from build123d import *

# Parameters (mm, degrees)
F0_R     = 5.5
F0_R_2   = 4.1
F1_DEPTH = 16
F0_R_3   = 2.55
F2_DEPTH = 5
F3_SIZE  = 1
F4_R     = 0.75


with BuildPart() as f1:
    # F0 (on Top) → F1 (new body)
    with BuildSketch(Plane.XY):
        Circle(F0_R)
        Circle(F0_R_2, mode=Mode.SUBTRACT)
    extrude(amount=F1_DEPTH)

    # F0 (on Top) → F2 (join)
    with BuildSketch(Plane.XY):
        Circle(F0_R_2)
        Circle(F0_R_3, mode=Mode.SUBTRACT)
    extrude(amount=F2_DEPTH)

    # F3
    f3_edges = [f1.edges().sort_by_distance(p)[0] for p in [
        (-5.5, 0, 0),
    ]]
    chamfer(f3_edges, length=F3_SIZE)

    # F4 (on Front) → F5 (revolve, cut)
    with BuildSketch(Plane.XZ):
        with Locations((5.526415, 5.650808)):
            Circle(F4_R)
    revolve(axis=Axis((0, 0, 0), (0, 0, -1)), mode=Mode.SUBTRACT)


solid = f1.part
Check sheet for the modelled part. Datum: model origin and axes. Units: mm. A direction names the side the tool comes from. Give positions to 0.01 mm unless a question says otherwise; leave off trailing zeros. Loops run counter-clockwise (first coordinate to the right, second up) from the corner with the lowest first, then second, coordinate; pieces in that order, holes last. Notation, with made-up numbers: M 34.25,84.5 L 43.25,84.5 A29 ccw 43.25,118.5 Z; hole C 25.25,55 d7. An arc over 180 degrees is marked long. Return JSON: item names as keys, results as strings. Group by question number.
1. Cross-section at D-D on z = 6. Record the boundary of the cut face in (x, y), plus the area to 3 significant figures.
2. Tool access check on faces 4 (the cylindrical face through (-1.19, -5.37, 2.92)), 5 (the flat face through (-2, -2, 5)). Record the directions out of +Z, -Z, +X, -X, +Y, -Y that give a thin tool (end or side, any length) a straight path to the whole face; none if there is none.
3. Mould release check, pull along Y, two halves, no side actions. Record for faces 1 (the cylindrical face through (-1.19, -5.37, 11.13)), 2 (the cylindrical face through (-0.534, 4.065, 10.423)), 3 (the flat face through (2, -2, 0)): released by +Y, released by -Y, zero draft, split by the parting line, or undercut.
4. Cross-section at A-A on y = 0. Record the boundary of the cut face in (x, z).
5. Thickness scan on L1, parallel to Y at x = 0, z = 9.5; L2, parallel to Y at x = 0, z = 1.6; L3, parallel to Z at x = 4.5, y = 3. Record the ranges inside material, lowest first.
6. Cross-section at C-C on z = 14.25. Record the boundary of the cut face in (x, y).
7. Go/stop test with flat-tipped pins: pin 1 (5 mm diameter, centred on x = 0, y = 0, fed in from +Z); pin 2 (6 mm diameter, centred on y = 3.5, z = 2, fed in from -X); pin 3 (4 mm diameter, centred on x = -3.5, z = 9.5, fed in from +Y). Record where each tip stops, or that it passes through.
Return value:
{
 "1": {"outline": "C 0,0 d9.73; hole C 0,0 d8.2", "area": "21.5 mm^2"},
 "2": {"face 4": "+Z, -Z", "face 5": "+Z"},
 "3": {"face 1": "split by the parting line", "face 2": "undercut", "face 3": "zero draft"},
 "4": {"outline": "M -5.5,1 L -4.5,0 L -2.55,0 L -2.55,5 L -4.1,5 L -4.1,16 L -5.5,16 L -5.5,6.4 A0.75 cw -5.5,4.9 Z; M 2.55,0 L 4.5,0 L 5.5,1 L 5.5,4.9 A0.75 cw 5.5,6.4 L 5.5,16 L 4.1,16 L 4.1,5 L 2.55,5 Z"},
 "5": {"L1": "-5.5 to -4.1, 4.1 to 5.5", "L2": "-5.5 to -2.55, 2.55 to 5.5", "L3": "0.91 to 4.91, 6.39 to 16"},
 "6": {"outline": "C 0,0 d11; hole C 0,0 d8.2"},
 "7": {"pin 1": "through", "pin 2": "x = -5.48", "pin 3": "y = 5.29"}
}
